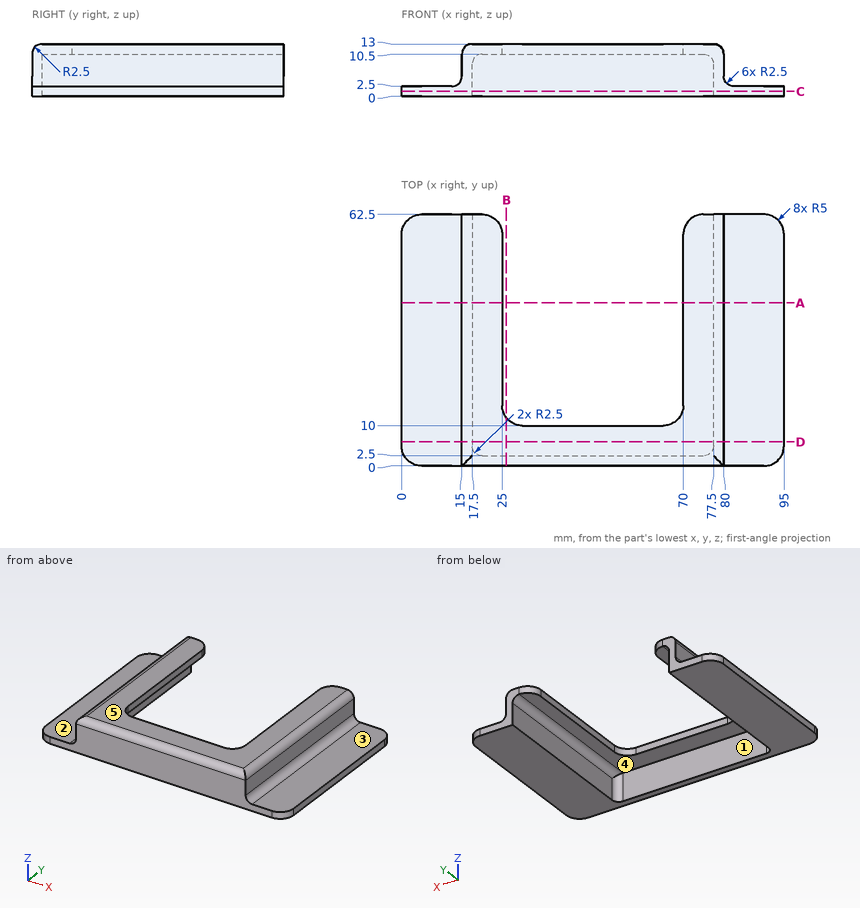
Check sheet for the drawn part. Datum: minimum x, y, z corner. Units: mm. A direction names the side the tool comes from. Give positions to 0.01 mm unless a question says otherwise; leave off trailing zeros. Write each loop counter-clockwise with the first axis right and the second up, starting at its lowest first coordinate (ties: lowest second). Pieces come first, ordered by that corner, then holes. Notation, with made-up numbers: (-39, -39) -> (-27, -39) arc R16 ccw to (-27, -19) -> close; hole circle Ø8 at (85.25, 20.25). An arc over 180 degrees is marked (long way). Use one line per item in the form item = value. Start each with the question number.
1. Section check C-C (z = 1.25). Record the cut outline in (x, y), and give its area (3 significant figures).
2. Go/stop test with flat-tipped pins: P1, Ø1.6, axis at y = 25.5, z = 9, coming from the -X side; P2, Ø1.5, axis at y = 47, z = 5, coming from the -X side; P3, Ø6.5, axis at y = 32, z = 2, coming from the -X side; P4, Ø4, axis at x = 87, y = 25, coming from the +Z side. Record where each tip stops, or that it passes through.
3. Thickness scan on line 1 along X through (y, z) = (8, 2.25); line 2 along X through (y, z) = (10, 7.75); line 3 along Y through (x, z) = (39, 9.75). Record the ranges inside material, lowest first. Write a range as from..to.
4. Mould release check, pull along X, two halves, no side actions. Record for the marked faces 4 and 5: pulls with the +X half, pulls with the -X half, needs draft (parallel to the pull), parting line crosses it, or undercut.
5. Section check A-A (y = 40.5). Record the cut outline in (x, z).
6. Section check D-D (y = 6). Record the cut outline in (x, z), and give its area (3 significant figures).
7. Section check B-B (x = 26). Record the cut outline in (y, z), and give its area (3 significant figures).
8. Access from +Z, -Z, +X, -X, +Y, -Y to the whole of each face (thin tool, end or side, straight path). Record for the marked faces 1, 2 and 3.
Conclusion:
q1.outline = (0, 5) arc R5 ccw to (5, 0) -> (90, 0) arc R5 ccw to (95, 5) -> (95, 57.5) arc R5 ccw to (90, 62.5) -> (77.5, 62.5) -> (77.5, 5) arc R2.5 cw to (75, 2.5) -> (20, 2.5) arc R2.5 cw to (17.5, 5) -> (17.5, 62.5) -> (5, 62.5) arc R5 ccw to (0, 57.5) -> close
q1.area = 2,320 mm²
q2.P1 = 15
q2.P2 = 14.88
q2.P3 = 0
q2.P4 = 2.5
q3.line_1 = 0..17.5, 77.5..95
q3.line_2 = 15..17.5, 77.5..80
q3.line_3 = 0..2.5
q4.face_4 = undercut
q4.face_5 = needs draft
q5.outline = (0, 0) -> (17.5, 0) -> (17.5, 8) arc R2.5 cw to (20, 10.5) -> (25, 10.5) -> (25, 13) -> (17.5, 13) arc R2.5 ccw to (15, 10.5) -> (15, 5) arc R2.5 cw to (12.5, 2.5) -> (0, 2.5) -> close; (70, 10.5) -> (75, 10.5) arc R2.5 cw to (77.5, 8) -> (77.5, 0) -> (95, 0) -> (95, 2.5) -> (82.5, 2.5) arc R2.5 cw to (80, 5) -> (80, 10.5) arc R2.5 ccw to (77.5, 13) -> (70, 13) -> close
q6.outline = (0, 0) -> (17.5, 0) -> (17.5, 8) arc R2.5 cw to (20, 10.5) -> (75, 10.5) arc R2.5 cw to (77.5, 8) -> (77.5, 0) -> (95, 0) -> (95, 2.5) -> (82.5, 2.5) arc R2.5 cw to (80, 5) -> (80, 10.5) arc R2.5 ccw to (77.5, 13) -> (17.5, 13) arc R2.5 ccw to (15, 10.5) -> (15, 5) arc R2.5 cw to (12.5, 2.5) -> (0, 2.5) -> close
q6.area = 293 mm²
q7.outline = (0, 0) -> (2.5, 0) -> (2.5, 10.5) -> (12, 10.5) -> (12, 13) -> (2.5, 13) arc R2.5 ccw to (0, 10.5) -> close
q7.area = 54.9 mm²
q8.face_1 = -Z, +Y
q8.face_2 = +Z, -X, +Y, -Y
q8.face_3 = +Z, +X, +Y, -Y
